Work out the finished part from the listing and answer in its coordinate system (mm). A direction names the side the tool comes from. Round coordinates to 2 decimals unless told otherwise and drop trailing zeros. Write each loop counter-clockwise with the first axis right and the second up, starting at its lowest first coordinate (ties: lowest second). Pieces come first, ordered by that corner, then holes. Notation, with made-up numbers: (-2, -6.75) -> (4, -6.75) arc R20 ccw to (4, -0.75) -> close; hole circle Ø7 at (-17.5, 20.5). An arc over 180 degrees is marked (long way). One line per item, written item: value.
```python
from build123d import *

# Parameters (mm, degrees)
SKETCH1_W            = 30.15
SKETCH1_H            = 30.15
BOSS_EXTRUDE1_DEPTH  = 7.75
FILLET1_R            = 3
M3_CLEARANCE_HOLE1_D = 3.2
SKETCH4_R            = 2.375
CUT_EXTRUDE1_DEPTH   = 3.25
SKETCH5_R            = 14.2
SKETCH5_R_2          = 8.6
CUT_EXTRUDE2_DEPTH   = 6.5


with BuildPart() as part:
    # Sketch1 → Boss-Extrude1 (new body)
    with BuildSketch(Plane(origin=(0, 0, 0), x_dir=(1, 0, 0), z_dir=(0, 1, 0))):
        Rectangle(SKETCH1_W, SKETCH1_H)
    extrude(amount=BOSS_EXTRUDE1_DEPTH)

    # Fillet1
    fillet1_edges = [part.edges().sort_by_distance(p)[0] for p in [
        (15.075, 3.875, 15.075),
        (-15.075, 3.875, 15.075),
        (-15.075, 3.875, -15.075),
        (15.075, 3.875, -15.075),
    ]]
    fillet(fillet1_edges, radius=FILLET1_R)

    # M3 Clearance Hole1 (through all)
    with Locations(Plane(origin=(0, 7.75, 0), x_dir=(1, 0, 0), z_dir=(0, 1, 0))):
        with Locations((-12.075, 12.075), (12.075, 12.075), (12.075, -12.075), (-12.075, -12.075)):
            Hole(M3_CLEARANCE_HOLE1_D / 2)

    # Sketch4 → Cut-Extrude1 (cut)
    with BuildSketch(Plane(origin=(0, 7.75, 0), x_dir=(1, 0, 0), z_dir=(0, 1, 0))):
        with Locations(Location((-12.075, 12.075, 0), (0, 0, 270))):
            Circle(SKETCH4_R)
        with Locations(Location((12.075, 12.075, 0), (0, 0, 270))):
            Circle(SKETCH4_R)
        with Locations(Location((-12.075, -12.075, 0), (0, 0, 270))):
            Circle(SKETCH4_R)
        with Locations(Location((12.075, -12.075, 0), (0, 0, 270))):
            Circle(SKETCH4_R)
    extrude(amount=-CUT_EXTRUDE1_DEPTH, mode=Mode.SUBTRACT)

    # Sketch5 → Cut-Extrude2 (cut)
    with BuildSketch(Plane(origin=(0, 7.75, 0), x_dir=(1, 0, 0), z_dir=(0, 1, 0))):
        with Locations(Location((0, 0, 0), (0, 0, 270))):
            Circle(SKETCH5_R)
        with Locations(Location((0, 0, 0), (0, 0, 270))):
            Circle(SKETCH5_R_2, mode=Mode.SUBTRACT)
    extrude(amount=-CUT_EXTRUDE2_DEPTH, mode=Mode.SUBTRACT)


solid = part.part
```
(1) Consider probe 1 along X at (y, z) = (5, 0) (3 decimals); probe 2 along Z at (x, y) = (6.5, 3.5) (3 decimals); probe 3 along Z at (x, y) = (-4, 5) (3 decimals). Determine where each line is inside the solid, lowest interval first.
Reported:
probe 1: x = -15.075 to -14.2, -8.6 to 8.6, 14.2 to 15.075
probe 2: z = -15.075 to -12.625, -5.631 to 5.631, 12.625 to 15.075
probe 3: z = -15.075 to -13.625, -7.613 to 7.613, 13.625 to 15.075
(2) Flat-ended cylindrical pins translate along their axes: pin 1 Ø1 at (x, z) = (1, 10.5) entering from +Y; pin 2 Ø2.5 at (x, z) = (12.075, 12.075) entering from -Y; pin 3 Ø4.5 at (x, z) = (-12.075, -12.075) entering from +Y. Find the tip coordinate at first contact, or state that the pin passes through.
Reported:
pin 1: stops at y = 1.25
pin 2: passes through
pin 3: stops at y = 4.5
(3) Find section C-C on y = 2. Give the vertices of the cut face in (x, z) (3 decimals).
Reported:
outline: (-15.075, -12.075) arc R3 ccw to (-12.075, -15.075) -> (12.075, -15.075) arc R3 ccw to (15.075, -12.075) -> (15.075, 12.075) arc R3 ccw to (12.075, 15.075) -> (-12.075, 15.075) arc R3 ccw to (-15.075, 12.075) -> close; circle Ø17.2 at (0, 0); hole circle Ø28.4 at (0, 0); hole circle Ø3.2 at (-12.075, -12.075); hole circle Ø3.2 at (-12.075, 12.075); hole circle Ø3.2 at (12.075, -12.075); hole circle Ø3.2 at (12.075, 12.075)
(4) For a pull along Z with two mould halves and no side action, classify faces 1 (the face through (11.17, 6.15, -9.88)), 2 (the face through (14.22, 3.93, -14.17)), 3 (the face through (10.63, 6.15, 10.19)), 4 (the face through (0, 4, 15.075)) as pulls with the +Z half, pulls with the -Z half, needs draft (parallel to the pull), parting line crosses it, or undercut.
Reported:
face 1: undercut
face 2: pulls with the -Z half
face 3: undercut
face 4: pulls with the +Z half
(5) Find section D-D on z = 5. Give the vertices of the cut face in (x, y) (3 decimals), plus the area to 3 significant figures.
Reported:
outline: (-15.075, 0) -> (15.075, 0) -> (15.075, 7.75) -> (13.291, 7.75) -> (13.291, 1.25) -> (6.997, 1.25) -> (6.997, 7.75) -> (-6.997, 7.75) -> (-6.997, 1.25) -> (-13.291, 1.25) -> (-13.291, 7.75) -> (-15.075, 7.75) -> close
area: 152 mm2
(6) Find section A-A on y = 6.5. Give the vertices of the cut face in (x, z) (3 decimals), plus the area to 3 significant figures.
Reported:
outline: (-15.075, -12.075) arc R3 ccw to (-12.075, -15.075) -> (12.075, -15.075) arc R3 ccw to (15.075, -12.075) -> (15.075, 12.075) arc R3 ccw to (12.075, 15.075) -> (-12.075, 15.075) arc R3 ccw to (-15.075, 12.075) -> close; circle Ø17.2 at (0, 0); hole circle Ø4.75 at (-12.075, -12.075); hole circle Ø4.75 at (-12.075, 12.075); hole circle Ø28.4 at (0, 0); hole circle Ø4.75 at (12.075, -12.075); hole circle Ø4.75 at (12.075, 12.075)
area: 429 mm2
(7) A tool of negligible diameter and unlimited length cuts with its end or side. For faces 5 (the face through (12, 4.5, -14)), 6 (the face through (-14.22, 3.93, 14.17)), from which of +Z, -Z, +X, -X, +Y, -Y can it reach the whole face along a straight path? Write none if from no direction.
Reported:
face 5: +Y
face 6: +Z, -X, +Y, -Y
(8) Find section B-B on x = 0. Give the vertices of the cut face in (y, z) (3 decimals), plus the area to 3 significant figures.
Reported:
outline: (0, -15.075) -> (7.75, -15.075) -> (7.75, -14.2) -> (1.25, -14.2) -> (1.25, -8.6) -> (7.75, -8.6) -> (7.75, 8.6) -> (1.25, 8.6) -> (1.25, 14.2) -> (7.75, 14.2) -> (7.75, 15.075) -> (0, 15.075) -> close
area: 161 mm2
